```python
from build123d import *

# Parameters (mm, degrees)
EXTRU_MINCE1_DEPTH = 25
CONG_1_R           = 1


with BuildPart() as part:
    # Esquisse1 → Extru.-Mince1 (new body)
    with BuildSketch(Plane.XY):
        with BuildLine():
            Line((-32.373305915, 0), (-22.373305915, 0))
            ThreePointArc((-22.373305915, 0), (-20.959092353, 0.585786438), (-20.373305915, 2))
            Line((-20.373305915, 2), (-20.373305915, 36))
            ThreePointArc((-20.373305915, 36), (-19.787519478, 37.414213562), (-18.373305915, 38))
            Line((-18.373305915, 38), (11.626694085, 38))
            ThreePointArc((11.626694085, 38), (13.040907647, 37.414213562), (13.626694085, 36))
            Line((13.626694085, 36), (13.626694085, 2))
            ThreePointArc((13.626694085, 2), (14.212480522, 0.585786438), (15.626694085, 0))
            Line((15.626694085, 0), (25.626694085, 0))
            Line((25.626694085, 0), (25.626694085, 2))
            Line((25.626694085, 2), (15.626694085, 2))
            Line((15.626694085, 2), (15.626694085, 36))
            ThreePointArc((15.626694085, 36), (14.455121209, 38.828427125), (11.626694085, 40))
            Line((11.626694085, 40), (-18.373305915, 40))
            ThreePointArc((-18.373305915, 40), (-21.20173304, 38.828427125), (-22.373305915, 36))
            Line((-22.373305915, 36), (-22.373305915, 2))
            Line((-22.373305915, 2), (-32.373305915, 2))
            Line((-32.373305915, 2), (-32.373305915, 0))
        make_face()
    extrude(amount=EXTRU_MINCE1_DEPTH)

    # Congé1
    cong_1_edges = [part.edges().sort_by_distance(p)[0] for p in [
        (-22.373305915, 2, 12.5),
        (15.626694085, 2, 12.5),
    ]]
    fillet(cong_1_edges, radius=CONG_1_R)


solid = part.part
```
Read the model definition and answer for the solid it produces. Units are mm, in the model's axes. A direction names the side the tool comes from. Coordinates: 2 decimals unless noted, no trailing zeros. Loops run counter-clockwise (first coordinate to the right, second up) from the corner with the lowest first, then second, coordinate; pieces in that order, holes last. Notation, with made-up numbers: (5, 74) - (62, 74) arc R22 cw to (62, 112) - close; hole circle Ø2 at (-27.5, 24). An arc over 180 degrees is marked (long way). Answer in a Markdown table with one row per item.
1. Determine the mould class of faces 1 (the face through (21, 0, 12)), 2 (the face through (-32.373, 1, 12)), 3 (the face through (-19.8, 37.4, 12.3)) for opening direction X: +X half, -X half, draft (parallel to the pull), parting line (faces both ways), or undercut.
Conclusion:
| item | result |
|---|---|
| face 1 | draft |
| face 2 | -X half |
| face 3 | undercut |
2. Find section D-D, the plane x = -19.5. Write down the section's boundary in (y, z), then the cut area to 3 significant figures.
Conclusion:
| item | result |
|---|---|
| outline | (37.65, 0) - (39.84, 0) - (39.84, 25) - (37.65, 25) - close |
| area | 54.6 mm² |
3. Straight lines are drawn through the part: line 1 (X direction, y = 3, z = 5); line 2 (Y direction, x = -25, z = 10.5); line 3 (Y direction, x = 6, z = 7.5). For each, find the intervals that lie inside material, in ascending order.
Conclusion:
| item | result |
|---|---|
| line 1 | x = -22.37 to -20.37, 13.63 to 15.63 |
| line 2 | y = 0 to 2 |
| line 3 | y = 38 to 40 |
4. Find section A-A, the plane y = 25. Write down the section's boundary in (x, z), then the cut area to 3 significant figures.
Conclusion:
| item | result |
|---|---|
| outline | (-22.37, 0) - (-20.37, 0) - (-20.37, 25) - (-22.37, 25) - close; (13.63, 0) - (15.63, 0) - (15.63, 25) - (13.63, 25) - close |
| area | 100 mm² |
5. Find section B-B, the plane z = 17.75. Write down the section's boundary in (x, y), then the cut area to 3 significant figures.
Conclusion:
| item | result |
|---|---|
| outline | (-32.37, 0) - (-22.37, 0) arc R2 ccw to (-20.37, 2) - (-20.37, 36) arc R2 cw to (-18.37, 38) - (11.63, 38) arc R2 cw to (13.63, 36) - (13.63, 2) arc R2 ccw to (15.63, 0) - (25.63, 0) - (25.63, 2) - (16.63, 2) arc R1 cw to (15.63, 3) - (15.63, 36) arc R4 ccw to (11.63, 40) - (-18.37, 40) arc R4 ccw to (-22.37, 36) - (-22.37, 3) arc R1 cw to (-23.37, 2) - (-32.37, 2) - close |
| area | 262 mm² |
6. Given pin 1 (12.5 mm diameter, centred on y = 24.5, z = 13.5, fed in from +X); pin 2 (8 mm diameter, centred on x = -26, z = 12, fed in from +Y); pin 3 (4.5 mm diameter, centred on x = 20.5, z = 16.5, fed in from +Y), each flat-ended and moving along its own axis, determine where each tip first touches the part or whether it passes through.
Conclusion:
| item | result |
|---|---|
| pin 1 | stops at x = 15.63 |
| pin 2 | stops at y = 37.69 |
| pin 3 | stops at y = 2 |
7. Which of the six approach directions +Z, -Z, +X, -X, +Y, -Y give full straight-line access (tool end or side, diameter ignored) to faces 4 (the face through (15.627, 19, 12)), 5 (the face through (-22.373, 20, 12)), 6 (the face through (13.627, 19, 12))?
Conclusion:
| item | result |
|---|---|
| face 4 | +Z, -Z, +X, +Y |
| face 5 | +Z, -Z, -X, +Y |
| face 6 | +Z, -Z, -Y |
8. Find section C-C, the plane x = -4. Write down the section's boundary in (y, z), then the cut area to 3 significant figures.
Conclusion:
| item | result |
|---|---|
| outline | (38, 0) - (40, 0) - (40, 25) - (38, 25) - close |
| area | 50.0 mm² |
